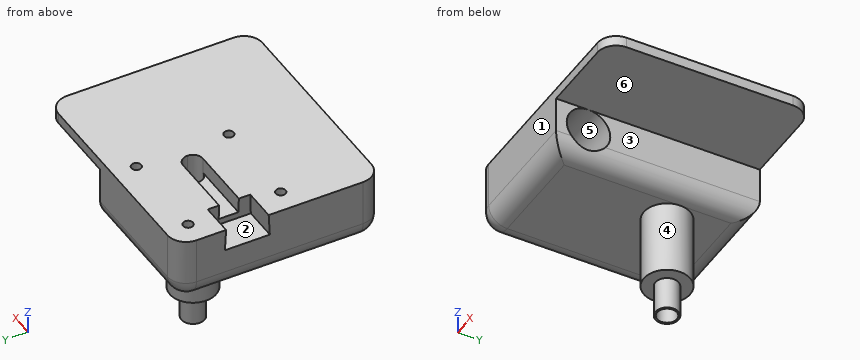
```python
from build123d import *
from build123d import SkipClean  # not in build123d's __all__

# Parameters (mm, degrees)
F0_W          = 38.1
F0_H          = 12.7
F1_DEPTH      = 19.05
F2_W          = 9.017
F2_H          = 3.1369
F2_H_2        = 5.4102
F3_DEPTH      = 6.096
F3_TAPER      = -3
F4_DEPTH      = 4.318
F5_DEPTH      = 12.7010001
F7_R          = 6.35
F7_R_2        = 2.7051
F8_DEPTH      = 25.4
F9_R          = 3.175
F9_R_2        = 2.7051
F10_DEPTH     = 9.017
F11_DEPTH     = 17.78
F12_DEPTH     = 5.08
F14_D         = 11.938
F14_DEPTH     = 25.4
F14_TIP       = 3.586537035
F15_W         = 55.88
F15_H         = 2.921
F16_DEPTH     = 25.4
F17_T1_DEPTH  = 25.4
F17_T3_DEPTH  = 28.321
F17_T5_DEPTH  = 45.72
F17_T7_DEPTH  = 45.72
F17_T9_DEPTH  = 81.28
F17_S13_W     = 5.08
F17_S13_H     = 5.08
F17_T14_DEPTH = 5.08
F17_S19_W     = 5.08
F17_S19_H     = 5.08
F17_T20_DEPTH = 5.08
F18_D         = 2.7051
F18_DEPTH     = 10.16
F18_TIP       = 0.8126940303


# Not quite as in the source:
# - a fillet or chamfer that OpenCascade refuses, or shapes differently, is made with other operations: its cross-section is extruded or revolved along the edge and cut away or added
# - after a boolean that leaves OpenCascade's solid faulty, fix() repairs it


with BuildPart() as f1:
    # F0 (on Front) → F1 (new body, symmetric)
    with BuildSketch(Plane.XZ):
        Rectangle(F0_W, F0_H)
    extrude(amount=F1_DEPTH, both=True)

    # F2 (on face) → F3 (cut)
    with BuildSketch(Plane.XY.offset(6.35)):
        with Locations((-14.5415, 4.27355)):
            Rectangle(F2_W, F2_H)
        with Locations((-14.5415, 0)):
            Rectangle(F2_W, F2_H_2)
        with Locations((-14.5415, -4.27355)):
            Rectangle(F2_W, F2_H)
    extrude(amount=-F3_DEPTH, taper=F3_TAPER, mode=Mode.SUBTRACT)

    # F2 (on face) → F4 (cut)
    with BuildSketch(Plane.XY.offset(6.35)):
        with Locations((-14.5415, 4.27355)):
            Rectangle(F2_W, F2_H)
        with Locations((-14.5415, -4.27355)):
            Rectangle(F2_W, F2_H)
        with BuildLine():
            Line((7.62, 2.7051), (1.8750079208, 2.7051))
            ThreePointArc((1.8750079208, 2.7051), (1.27, 0), (1.8750079208, -2.7051))
            Line((1.8750079208, -2.7051), (7.62, -2.7051))
            ThreePointArc((7.62, -2.7051), (4.9149, 0), (7.62, 2.7051))
        make_face()
        with BuildLine():
            ThreePointArc((1.8750079208, -2.7051), (1.27, 0), (1.8750079208, 2.7051))
            Line((1.8750079208, 2.7051), (-10.033, 2.7051))
            Line((-10.033, 2.7051), (-10.033, -2.7051))
            Line((-10.033, -2.7051), (1.8750079208, -2.7051))
        make_face()
        with Locations((-14.5415, 0)):
            Rectangle(F2_W, F2_H_2)
    extrude(amount=-F4_DEPTH, mode=Mode.SUBTRACT)

    # F2 (on face) → F5 (cut, through all)
    with BuildSketch(Plane.XY.offset(6.35)):
        with BuildLine():
            ThreePointArc((10.3251, 0), (9.5327945538, 1.9127945538), (7.62, 2.7051))
            ThreePointArc((7.62, 2.7051), (4.9149, 0), (7.62, -2.7051))
            ThreePointArc((7.62, -2.7051), (9.5327945538, -1.9127945538), (10.3251, 0))
        make_face()
    extrude(amount=-F5_DEPTH, mode=Mode.SUBTRACT)

    # F7 (on face) → F8 (join)
    with BuildSketch(Plane(origin=(0, 0, -6.35), x_dir=(1, 0, 0), z_dir=(0, 0, -1))):
        with Locations((7.62, 0)):
            Circle(F7_R)
        with Locations((7.62, 0)):
            Circle(F7_R_2, mode=Mode.SUBTRACT)
    with SkipClean():  # cleaning this boolean's faces spoils the solid; the shape is the same uncleaned
        extrude(amount=F8_DEPTH)

    # F9 (on face) → F10 (join)
    with BuildSketch(Plane(origin=(0, 0, -31.75), x_dir=(1, 0, 0), z_dir=(0, 0, -1))):
        with Locations((7.62, 0)):
            Circle(F9_R)
        with Locations((7.62, 0)):
            Circle(F9_R_2, mode=Mode.SUBTRACT)
    extrude(amount=F10_DEPTH)

    add(f1.part.fix(), mode=Mode.REPLACE)

    # F11 (add): a face of the model
    f11_faces = [f1.faces().sort_by_distance(p)[0] for p in [
        (0, -19.05, 0),
    ]]
    extrude(f11_faces, amount=F11_DEPTH)

    # F12 (add): faces of the model
    f12_faces = [f1.faces().sort_by_distance(p)[0] for p in [
        (-0.7285482759, 0, -6.35),
        (0, -27.94, -6.35),
    ]]
    extrude(f12_faces, amount=F12_DEPTH)

    # F14
    with Locations(Plane.YZ.offset(19.05)):
        with Locations((-27.94, -2.54)):
            Hole(F14_D / 2, depth=F14_DEPTH)
            with Locations((0, 0, -(F14_DEPTH + F14_TIP / 2))):  # 118° drill point
                Cone(0, F14_D / 2, F14_TIP, mode=Mode.SUBTRACT)

    # F15 (on face) → F16 (join)
    with BuildSketch(Plane.YZ.offset(19.05)):
        with Locations((-8.89, 4.8895)):
            Rectangle(F15_W, F15_H)
    extrude(amount=F16_DEPTH)

    # F17: fillet of radius 5.08 on 8 edges, made by hand

    # F17_s2 → F17_t1 (cut)
    with BuildSketch(Plane.XY.offset(-6.35)):
        with BuildLine():
            ThreePointArc((-13.97, -36.83), (-17.5621024484, -35.3421024484), (-19.05, -31.75))
            Line((-19.05, -31.75), (-19.05, -36.83))
            Line((-19.05, -36.83), (-13.97, -36.83))
        make_face()
        with BuildLine():
            ThreePointArc((-13.97, 19.05), (-17.5621024484, 17.5621024484), (-19.05, 13.97))
            Line((-19.05, 13.97), (-19.05, 19.05))
            Line((-19.05, 19.05), (-13.97, 19.05))
        make_face()
    extrude(amount=F17_T1_DEPTH, mode=Mode.SUBTRACT)

    # F17_s4 → F17_t3 (cut)
    with BuildSketch(Plane.XY.offset(-9.271)):
        with BuildLine():
            ThreePointArc((39.37, 19.05), (42.9621024484, 17.5621024484), (44.45, 13.97))
            Line((44.45, 13.97), (44.45, 19.05))
            Line((44.45, 19.05), (39.37, 19.05))
        make_face()
        with BuildLine():
            ThreePointArc((44.45, -31.75), (42.9621024484, -35.3421024484), (39.37, -36.83))
            Line((39.37, -36.83), (44.45, -36.83))
            Line((44.45, -36.83), (44.45, -31.75))
        make_face()
    extrude(amount=F17_T3_DEPTH, mode=Mode.SUBTRACT)

    # F17_s6 → F17_t5 (cut)
    with BuildSketch(Plane.XZ.offset(-13.97)):
        with BuildLine():
            ThreePointArc((-13.97, -11.43), (-17.5621024484, -9.9421024484), (-19.05, -6.35))
            Line((-19.05, -6.35), (-19.05, -11.43))
            Line((-19.05, -11.43), (-13.97, -11.43))
        make_face()
    extrude(amount=F17_T5_DEPTH, mode=Mode.SUBTRACT)

    # F17_s8 → F17_t7 (cut)
    with BuildSketch(Plane.YZ.offset(-13.97)):
        with BuildLine():
            ThreePointArc((-31.75, -11.43), (-35.3421024484, -9.9421024484), (-36.83, -6.35))
            Line((-36.83, -6.35), (-36.83, -11.43))
            Line((-36.83, -11.43), (-31.75, -11.43))
        make_face()
        with BuildLine():
            ThreePointArc((13.97, -11.43), (17.5621024484, -9.9421024484), (19.05, -6.35))
            Line((19.05, -6.35), (19.05, -11.43))
            Line((19.05, -11.43), (13.97, -11.43))
        make_face()
    extrude(amount=F17_T7_DEPTH, mode=Mode.SUBTRACT)

    # F17_s10 → F17_t9 (cut)
    with BuildSketch(Plane.XZ.offset(-31.75)):
        with BuildLine():
            ThreePointArc((13.97, -11.43), (17.5621024484, -9.9421024484), (19.05, -6.35))
            Line((19.05, -6.35), (19.05, -11.43))
            Line((19.05, -11.43), (13.97, -11.43))
        make_face()
    extrude(amount=F17_T9_DEPTH, mode=Mode.SUBTRACT)


with BuildPart() as f17_tool12:
    # F17_s13 → F17_t14 (new body)
    with BuildSketch(Plane.XY.offset(-6.35)):
        with Locations((-16.51, -34.29)):
            Rectangle(F17_S13_W, F17_S13_H)
    extrude(amount=-F17_T14_DEPTH)

    # F17_s15 → F17_t16 (revolve, cut)
    with BuildSketch(Plane(origin=(-13.97, -31.75, -6.35), x_dir=(0.7071067812, 0.7071067812, 0), z_dir=(-0.7071067812, 0.7071067812, 0))):
        with BuildLine():
            ThreePointArc((0, -5.08), (5.08, 0), (0, 5.08))
            Line((0, 5.08), (0, -5.08))
        make_face()
    revolve(axis=Axis((-13.97, -31.75, -6.35), (0, 0, -1)), mode=Mode.SUBTRACT)


with BuildPart() as f1_1:
    add(f1.part, clean=False)

    # F17_t11: cut F17_tool12
    add(f17_tool12.part, mode=Mode.SUBTRACT)


with BuildPart() as f17_tool18:
    # F17_s19 → F17_t20 (new body)
    with BuildSketch(Plane.XZ.offset(-13.97)):
        with Locations((-16.51, -8.89)):
            Rectangle(F17_S19_W, F17_S19_H)
    extrude(amount=-F17_T20_DEPTH)

    # F17_s21 → F17_t22 (revolve, cut)
    with BuildSketch(Plane(origin=(-13.97, 13.97, -6.35), x_dir=(0.7071067812, 0, 0.7071067812), z_dir=(-0.7071067812, 0, 0.7071067812))):
        with BuildLine():
            ThreePointArc((0, -5.08), (5.08, 0), (0, 5.08))
            Line((0, 5.08), (0, -5.08))
        make_face()
    revolve(axis=Axis((-13.97, 13.97, -6.35), (0, 1, 0)), mode=Mode.SUBTRACT)


with BuildPart() as f1_2:
    add(f1_1.part, clean=False)

    # F17_t17: cut F17_tool18
    add(f17_tool18.part, mode=Mode.SUBTRACT)

    # F18
    with Locations(Plane.XY.offset(6.35)):
        with Locations((-12.7, 12.7), (-12.7, -12.7), (12.7, -12.7), (12.7, 12.7)):
            Hole(F18_D / 2, depth=F18_DEPTH)
            with Locations((0, 0, -(F18_DEPTH + F18_TIP / 2))):  # 118° drill point
                Cone(0, F18_D / 2, F18_TIP, mode=Mode.SUBTRACT)


solid = f1_2.part
```
Geometry check sheet. Reference: the model listing, model coordinates, mm. Face numbers are marked on the shaded views. A direction names the side the tool comes from. Coordinates: 2 decimals unless noted, no trailing zeros. Write each loop counter-clockwise with the first axis right and the second up, starting at its lowest first coordinate (ties: lowest second). Pieces come first, ordered by that corner, then holes. Notation, with made-up numbers: M 0,-33 L 28,-33 A3 cw 28,-29 Z; hole C 66,54.25 d8. An arc over 180 degrees is marked long. One line per item, written item: value. Start each with the question number.
(1) Sectioned sample at A-A, the plane x = -3. Enter the section's corners in (y, z).
(2) Release check for a two-part mould opening along Y. For the marked faces 1, 2 and 3 record: released by +Y, released by -Y, zero draft, split by the parting line, or undercut.
(3) Scan lines: line 1 along Y through (x, z) = (-12.7, 0.5); line 2 along X through (y, z) = (-12.7, 2); line 3 along X through (y, z) = (0, -23). Record each from-to range of solid material in increasing order. Write a range as [from, to].
(4) Sectioned sample at B-B, the plane z = -29.5. Enter the section's corners in (x, y), and give its area (3 significant figures).
(5) Depth check by flat-ended pin: pin 1 (3 mm diameter, centred on x = -16.5, y = -2.5, fed in from +Z); pin 2 (6 mm diameter, centred on x = 7.62, y = 0, fed in from -Z); pin 3 (3.5 mm diameter, centred on x = 12.7, y = -12.7, fed in from -Z); pin 4 (20.5 mm diameter, centred on x = 34, y = -8, fed in from -Z). Enter the tip coordinate at first touch or a pass-through.
(6) Sectioned sample at C-C, the plane x = 35.5. Enter the section's corners in (y, z), and give its area (3 significant figures).
(7) Tool access check on the marked faces 4, 5 and 6. Record the directions out of +Z, -Z, +X, -X, +Y, -Y that give a thin tool (end or side, any length) a straight path to the whole face; none if there is none.
Filled sheet:
1. outline: M -36.83,-6.35 A5.08 ccw -31.75,-11.43 L 13.97,-11.43 A5.08 ccw 19.05,-6.35 L 19.05,6.35 L 2.71,6.35 L 2.71,2.03 L -2.71,2.03 L -2.71,6.35 L -36.83,6.35 Z; hole C -27.94,-2.54 d11.94
2. face 1: released by -Y
2. face 2: undercut
2. face 3: zero draft
3. line 1: [-36.83, -14.05], [-11.35, -6.15], [6.15, 11.35], [14.05, 19.05]
3. line 2: [-19.05, -14.05], [-11.35, 11.35], [14.05, 19.05]
3. line 3: [1.27, 4.91], [10.33, 13.97]
4. outline: C 7.62,0 d12.7; hole C 7.62,0 d5.41
4. area: 104 mm²
5. pin 1: z = 0.25
5. pin 2: z = -40.77
5. pin 3: z = -11.43
5. pin 4: z = 3.43
6. outline: M -36.83,3.43 L 19.05,3.43 L 19.05,6.35 L -36.83,6.35 Z
6. area: 163 mm²
7. face 4: -Z
7. face 5: +X
7. face 6: -Z, +X, +Y, -Y
